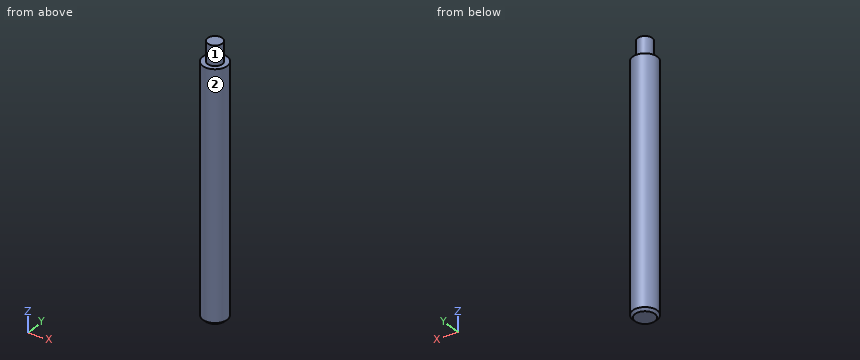
Autodesk Inventor part; units mm, degrees
ref_plane "YZ Plane" through (0, 0, 0) normal (1, 0, 0) x (0, 1, 0)
ref_plane "XZ Plane" through (0, 0, 0) normal (0, 1, 0) x (-1, 0, 0)
ref_plane "XY Plane" through (0, 0, 0) normal (0, 0, 1) x (1, 0, 0)
sketch "Sketch1" plane through (0, 0, 0) normal (0, 0, 1) x (1, 0, 0)
  circle A0 centre (0, 0) radius 5
  dimension "d0" = 10
extrude "Extrusion1" add sketch "Sketch1" along normal blind 100
sketch "Sketch3" plane through (0, 0, 100) normal (0, 0, 1) x (1, 0, 0)
  circle A0 centre (0, 0) radius 5
  circle A1 centre (0, 0) radius 3
  dimension "d3" = 6
extrude "Extrusion2" add sketch "Sketch3" along normal blind 8 contours A1
thread "Thread1"
chamfer "Chamfer1" distance 1 angle 45 1 edges at (-5, 0, 0)
properties part number "rod"
Input: part model. Units: mm. Frame: model coordinates. Face numbers are marked on the shaded views. A direction names the side the tool comes from. Coordinates: 2 decimals unless noted, no trailing zeros. Loops run counter-clockwise (first coordinate to the right, second up) from the corner with the lowest first, then second, coordinate; pieces in that order, holes last.
(1) Material intervals for probe 1 along X at (y, z) = (-0.25, 40.5); probe 2 along X at (y, z) = (-4, 33); probe 3 along Z at (x, y) = (0.75, 3.5), sorted ascending.
(2) Section C-C on z = 17.5. Return the cut outline in (x, y).
(3) Section A-A on y = 0. Return the cut outline in (x, z), then the cut area to 3 significant figures.
(4) First-contact query: pin 1 Ø1 at (x, z) = (-1, 68) entering from -Y; pin 2 Ø4 at (x, z) = (3.5, 95) entering from -Y; pin 3 Ø3 at (y, z) = (-3, 46.5) entering from -X. Flat tips, straight axial feed; report the tip coordinate or a pass-through.
(5) Set-up query: the marked faces 1 and 2. Return all of +Z, -Z, +X, -X, +Y, -Y with unobstructed straight access to the full face (end or side cutting, diameter ignored); none if empty.
Data:
1. probe 1: x = -4.99 to 4.99
1. probe 2: x = -3 to 3
1. probe 3: z = 0 to 100
2. outline: circle Ø10 at (0, 0)
3. outline: (-5, 1) - (-4, 0) - (4, 0) - (5, 1) - (5, 100) - (3, 100) - (3, 108) - (-3, 108) - (-3, 100) - (-5, 100) - close
3. area: 1,050 mm2
4. pin 1: stops at y = -4.97
4. pin 2: stops at y = -4.77
4. pin 3: stops at x = -4.77
5. face 1: +Z
5. face 2: +Z, -Z
